```python
from build123d import *

# Parameters (mm, degrees)
SALIENTE_EXTRUIR1_DEPTH = 3


with BuildPart() as part:
    # Model → Saliente-Extruir1 (new body)
    with BuildSketch(Plane.XY):
        with BuildLine():
            Line((-36.413611368, 21.5), (-36.413611368, 15.5))
            Line((-36.413611368, 15.5), (-36.413611368, 1.5))
            Line((-36.413611368, 1.5), (-37.413611368, 1.5))
            Line((-37.413611368, 1.5), (-37.413611368, -0.5))
            Line((-37.413611368, -0.5), (-38.413611368, -0.5))
            Line((-38.413611368, -0.5), (-38.413611368, -48.5))
            ThreePointArc((-38.413611368, -48.5), (-38.999397805, -49.914213562), (-40.413611368, -50.5))
            Line((-40.413611368, -50.5), (-41.413611368, -50.5))
            ThreePointArc((-41.413611368, -50.5), (-42.82782493, -49.914213562), (-43.413611368, -48.5))
            Line((-43.413611368, -48.5), (-43.413611368, -0.5))
            Line((-43.413611368, -0.5), (-44.413611368, -0.5))
            Line((-44.413611368, -0.5), (-44.413611368, 1.5))
            Line((-44.413611368, 1.5), (-45.413611368, 1.5))
            Line((-45.413611368, 1.5), (-45.413611368, 21.5))
            Line((-45.413611368, 21.5), (-36.413611368, 21.5))
        make_face()
    extrude(amount=SALIENTE_EXTRUIR1_DEPTH)


solid = part.part
```
Source: CAD feature listing. Evaluate the final solid. Frame: model axes, mm. A direction names the side the tool comes from. Coordinates: 2 decimals unless noted, no trailing zeros. Write each loop counter-clockwise with the first axis right and the second up, starting at its lowest first coordinate (ties: lowest second). Pieces come first, ordered by that corner, then holes. Notation, with made-up numbers: (43.25, 42.5) -> (48.25, 42.5) arc R32 cw to (48.25, 74.5) -> close; hole circle Ø4 at (84.5, 34.25). An arc over 180 degrees is marked (long way). Return JSON: item names as keys, results as strings. Group by question number.
1) Section query B-B, the plane y = -38. Return loops of the section in (x, z), plus the area to 3 significant figures.
2) Section query A-A, the plane z = 1.2. Return loops of the section in (x, y), plus the area to 3 significant figures.
3) Set-up query: faces 1 (the face through (-43.414, -25, 1)), 2 (the face through (-41, -6, 3)), 3 (the face through (-37.414, 1, 1)). Return all of +Z, -Z, +X, -X, +Y, -Y with unobstructed straight access to the full face (end or side cutting, diameter ignored); none if empty.
4) Contact query for flat-ended pins moving along their axis: P1, Ø0.5, axis at x = -38, z = 1, coming from the -Y side; P2, Ø1.1, axis at x = -45, z = 1.5, coming from the -Y side; P3, Ø0.9, axis at y = -22, z = 1.5, coming from the -X side. Output: stop coordinate, or through.
5) Ray query, line 1 along Y through (x, z) = (-37, 2); line 2 along Y through (x, z) = (-43.75, 0.45); line 3 along X through (y, z) = (-22, 1.05). Return the intervals inside material, ascending.
From the geometry:
{
 "1": {"outline": "(-43.41, 0) -> (-38.41, 0) -> (-38.41, 3) -> (-43.41, 3) -> close", "area": "15.0 mm²"},
 "2": {"outline": "(-45.41, 1.5) -> (-44.41, 1.5) -> (-44.41, -0.5) -> (-43.41, -0.5) -> (-43.41, -48.5) arc R2 ccw to (-41.41, -50.5) -> (-40.41, -50.5) arc R2 ccw to (-38.41, -48.5) -> (-38.41, -0.5) -> (-37.41, -0.5) -> (-37.41, 1.5) -> (-36.41, 1.5) -> (-36.41, 21.5) -> (-45.41, 21.5) -> close", "area": "442 mm²"},
 "3": {"face 1": "+Z, -Z, -X, -Y", "face 2": "+Z, +X, -X, +Y, -Y", "face 3": "+Z, -Z, +X, -Y"},
 "4": {"P1": "y = -0.5", "P2": "y = 1.5", "P3": "x = -43.41"},
 "5": {"line 1": "1.5 to 21.5", "line 2": "-0.5 to 21.5", "line 3": "-43.41 to -38.41"}
}
